Could you check a few things on this model? Use its own coordinates, in mm. A direction names the side the tool comes from. Give positions to 0.01 mm unless a question says otherwise; leave off trailing zeros. Order: outer loops, then holes, each group sorted by start corner. A loop starts at its lowest first (then second) coordinate and runs counter-clockwise, first axis right, second up. Notation, with made-up numbers: (58.25, -15.75) - (75.25, -15.75) arc R12 cw to (75.25, 6.25) - close; hole circle Ø11 at (-7.75, -39). An arc over 180 degrees is marked (long way). One line per question, with ' | ' between items. Start each with the question number.
1. Which directions (+Z, -Z, +X, -X, +Y, -Y) give clear straight access to the entire face, cutting with the end or side of a thin tool? Please do faces 4 (the flat face through (0, 11, -46)), 5 (the flat face through (-14, 20, -25.804)).
2. Imagine slicing it at B-B (z = -84.5). Please give me the cut outline in (x, y), and give its area (3 significant figures).
3. Imagine slicing it at D-D (z = -56). Please give me the cut outline in (x, y), and give its area (3 significant figures).
4. I need wall thicknesses on probe 1 along Z at (x, y) = (-7, 10.25); probe 2 along Z at (x, y) = (-7, 19.5); probe 3 along Z at (x, y) = (-14, 19). Which ranges of each line are inside material? Lowest first, please. Write a range as from..to.
5. Imagine slicing it at A-A (x = -6.25). Please give me the cut outline in (y, z), and give its area (3 significant figures).
6. If we mould it in two halves opening along Z, with no side actions, what happens to faces 1 (the cylindrical face through (-9.59, 24.1, -0.86)), 2 (the flat face through (-14, 5, -58)), 3 (the flat face through (-10, 0, -45))? For each: released by +Z, released by -Z, zero draft, split by the parting line, or undercut.
7. For P1, Ø1.5, axis at x = -5.5, z = -16, coming from the -Y side; P2, Ø1.2, axis at x = -14, z = -57.5, coming from the +Y side; P3, Ø3, axis at x = -7, z = -6.5, coming from the +Y side; P4, Ø9.5, axis at y = 16, z = -39.5, coming from the -X side, each with a flat end and sliding along its axis, tell me the tip position at first contact or that it passes through.
8. Imagine slicing it at C-C (y = 8.5). Please give me the cut outline in (x, z).
Autodesk Inventor part; units mm, degrees
ref_plane "YZ Plane" through (0, 0, 0) normal (1, 0, 0) x (0, 1, 0)
ref_plane "XZ Plane" through (0, 0, 0) normal (0, 1, 0) x (-1, 0, 0)
ref_plane "XY Plane" through (0, 0, 0) normal (0, 0, 1) x (1, 0, 0)
sketch "Sketch1" plane through (0, 0, 0) normal (0, 1, 0) x (-1, 0, 0)
  line L0 (0, 0) -> (16, 0)
  line L1 (16, 0) -> (16, -91)
  line L2 (16, -91) -> (0, -91)
  line L3 (0, -91) -> (0, 0)
  dimension "d0" = 16
  dimension "d1" = 91
extrude "Extrusion1" add sketch "Sketch1" along normal blind 25
sketch "Sketch2" plane through (0, 25, 0) normal (0, 1, 0) x (1, 0, 0)
  line L0 (-16, 91) -> (-16, 0)
  circle A0 centre (-16, 12.8045) radius 4
  circle A1 centre (-16, 57.8045) radius 4
  point P0 (0, 0)
  dimension "d4" = 8
  dimension "d5" = 8
  dimension "d6" = 45
extrude "Extrusion2" cut sketch "Sketch2" against normal blind 20
fillet "Fillet1" radius 3 5 edges at (0, 12.5, -91) (0, 12.5, 0) (0, 25, -45.5) (-8, 25, -91) (-8, 25, 0)
sketch "Sketch3" plane through (0, 25, 0) normal (0, 1, 0) x (1, 0, 0)
  circle A0 centre (-7, 6.5) radius 2
  circle A1 centre (-7, 45.5) radius 2
  circle A2 centre (-7, 84.5) radius 2
  line L0 (-16, 8.8045) -> (-16, 3)
  line L1 (-16, 53.8045) -> (-16, 16.8045)
  line L2 (-16, 88) -> (-16, 61.8045)
  point P0 (0, 0)
  dimension "d10" = 4
  dimension "d11" = 4
  dimension "d12" = 4
  dimension "d13" = 39
  dimension "d14" = 39
  dimension "d15" = 9
  dimension "d16" = 9
  dimension "d17" = 9
  dimension "d18" = 6.5
extrude "Extrusion3" cut sketch "Sketch3" against normal blind 30
sketch "Sketch4" plane through (0, 0, -3) normal (1, 0, 0) x (0, 0, -1)
  circle A0 centre (17.4261, 19.4387) radius 2
  circle A1 centre (69.9995, 19.4387) radius 2
  point P0 (-3, 0)
  dimension "d21" = 4
  dimension "d22" = 4
extrude "Extrusion4" cut sketch "Sketch4" against normal blind 30
sketch "Sketch5" plane through (-16, 0, -91) normal (-1, 0, 0) x (0, 0, 1)
  point P0 (91, 0)
sketch "Sketch6" plane through (-16, 0, -91) normal (-1, 0, 0) x (0, 0, 1)
  arc A0 (46.1955, 15) -> (65.1955, 15) centre (55.6955, 15) ccw
  line L0 (37.1955, 25) -> (37.1955, 5)
  line L1 (37.1955, 25) -> (74.1955, 25)
  line L2 (46.1955, 15) -> (46.1955, 30.0529)
  line L3 (46.1955, 30.0529) -> (65.1955, 30.0529)
  line L4 (65.1955, 30.0529) -> (65.1955, 15)
  point P0 (91, 0)
  dimension "d25" = 19
  dimension "d26" = 18.5
  dimension "d27" = 10
extrude "Extrusion5" cut sketch "Sketch6" against normal blind 4.5
sketch "Sketch7" plane through (-11.5, 0, -91) normal (-1, 0, 0) x (0, 0, 1)
  circle A0 centre (55.6955, 15) radius 2.75
  line L0 (37.1955, 25) -> (37.1955, 5)
  point P0 (91, 0)
  dimension "d30" = 5.5
  dimension "d31" = 18.5
extrude "Extrusion6" cut sketch "Sketch7" against normal blind 30
properties part number "ldlerradrod"
Results found:
1) face 4: +Z, -Z, +X, +Y, -Y | face 5: -X, +Y
2) outline: (-16, 0) - (-9, 0) - (-9, 25) - (-16, 25) - close; (-5, 0) - (0, 0) - (0, 22) arc R3 ccw to (-3, 25) - (-5, 25) - close | area: 298 mm2
3) outline: (-16, 0) - (0, 0) - (0, 22) arc R3 ccw to (-3, 25) - (-12.43, 25) - (-12.43, 5) - (-16, 5) - close | area: 327 mm2
4) probe 1: z = -91..-86.5, -82.5..-47.5, -43.5..-8.5, -4.5..0 | probe 2: z = -91..-86.5, -82.5..-75, -71..-47.5, -43.5..-22.43, -18.43..-8.5, -4.5..0 | probe 3: z = -91..-74.95, -71.05..-61.27, -54.34..-44.8, -25.8..-22.38, -18.47..-16.27, -9.34..0
5) outline: (0, -91) - (22, -91) arc R3 ccw to (25, -88) - (25, -86.35) - (0, -86.35) - close; (0, -82.65) - (25, -82.65) - (25, -47.35) - (0, -47.35) - close; (0, -43.65) - (25, -43.65) - (25, -8.35) - (0, -8.35) - close; (0, -4.65) - (25, -4.65) - (25, -3) arc R3 ccw to (22, 0) - (0, 0) - close; hole circle Ø5.5 at (15, -35.3); hole circle Ø4 at (19.44, -73); hole circle Ø4 at (19.44, -20.43) | area: 1,940 mm2
6) face 1: released by +Z | face 2: undercut | face 3: zero draft
7) P1: stops at y = 0 | P2: stops at y = 5 | P3: passes through | P4: stops at x = -11.5
8) outline: (-16, -91) - (-3, -91) arc R3 ccw to (0, -88) - (0, -3) arc R3 ccw to (-3, 0) - (-16, 0) - (-16, -8.8) arc R4 cw to (-16, -16.8) - (-16, -28.38) - (-11.5, -28.38) - (-11.5, -42.23) - (-16, -42.23) - (-16, -53.8) arc R4 cw to (-16, -61.8) - close; hole circle Ø4 at (-7, -84.5); hole circle Ø4 at (-7, -45.5); hole circle Ø4 at (-7, -6.5)
